from build123d import *

# Parameters (mm, degrees)
BOSS_EXTRUDE1_DEPTH = 55
SKETCH2_R           = 2.5
CUT_EXTRUDE1_DEPTH  = 2
SKETCH3_W           = 1
SKETCH3_H           = 9
CUT_EXTRUDE2_DEPTH  = 35
SKETCH4_R           = 2.25
CUT_EXTRUDE3_DEPTH  = 11


with BuildPart() as part:
    # Sketch1 → Boss-Extrude1 (new body)
    with BuildSketch(Plane.XY):
        Polygon((0, 10), (0, 0), (10, 0), (10, 1), (1, 1), (1, 10), align=None)
    extrude(amount=BOSS_EXTRUDE1_DEPTH)

    # Sketch2 → Cut-Extrude1 (cut, through all)
    with BuildSketch(Plane(origin=(0, 1, 0), x_dir=(1, 0, 0), z_dir=(0, 1, 0))):
        with Locations((5, -50)):
            Circle(SKETCH2_R)
        with Locations((5, -26.95)):
            Circle(SKETCH2_R)
        with BuildLine():
            Line((-2.7555139, -28.141028133), (-2.7555139, -48.808971867))
            ThreePointArc((-2.7555139, -48.808971867), (4.475, -38.475), (-2.7555139, -28.141028133))
        make_face()
    extrude(amount=-CUT_EXTRUDE1_DEPTH, mode=Mode.SUBTRACT)

    # Sketch3 → Cut-Extrude2 (cut)
    with BuildSketch(Plane.XY.offset(55)):
        with Locations((0.5, 5.5)):
            Rectangle(SKETCH3_W, SKETCH3_H)
    extrude(amount=-CUT_EXTRUDE2_DEPTH, mode=Mode.SUBTRACT)

    # Sketch4 → Cut-Extrude3 (cut, through all)
    with BuildSketch(Plane.ZY):
        with Locations((5.1, 4)):
            Circle(SKETCH4_R)
        with Locations((15.1, 4)):
            Circle(SKETCH4_R)
    extrude(amount=-CUT_EXTRUDE3_DEPTH, mode=Mode.SUBTRACT)


solid = part.part
The model under review builds one solid part; all positions refer to its coordinate system, in mm. A direction names the side the tool comes from. Round coordinates to 2 decimals unless told otherwise and drop trailing zeros. Loops run counter-clockwise (first coordinate to the right, second up) from the corner with the lowest first, then second, coordinate; pieces in that order, holes last. Notation, with made-up numbers: M 51.5,-1 L 69.5,-1 A19 cw 69.5,13 Z; hole C 72,33.5 d8. An arc over 180 degrees is marked long. Answer as CSV lines item,"result". Start each with the question number.
Item 1: Wall thickness on line 1 (X direction, y = 0.3, z = 26.95); line 2 (Z direction, x = 5, y = 0.55); line 3 (Y direction, x = 0.4, z = 5.1): over which ranges is each line inside the solid? List them lowest first. Write a range as [from, to].
Item 2: Consider section A-A (x = 5). Write out the cut boundary in (y, z).
Item 3: Insertion check: P1, Ø4.5, axis at x = 5, z = 50, coming from the -Y side; P2, Ø1.1, axis at x = 0.5, y = 6, coming from the +Z side. Each pin has a flat end and moves straight along its axis. Give the tip position at first contact, or say it passes through.
Item 4: Consider section B-B (z = 50). Write out the cut boundary in (x, y), then the cut area to 3 significant figures.
Item 5: For faces 4 (the face through (1, 5, 10)), 5 (the face through (0.5, 5.6, 20)), 6 (the face through (5, 0, 21)), list the 3-axis set-ups (+Z, -Z, +X, -X, +Y, -Y) from which the entire face can be reached by the end or side of a thin tool; tool diameter is ignored.
Item 6: Mouldability with a two-part tool opening along X and no side actions: class faces 1 (the face through (4.474, 0.507, 38.619)), 2 (the face through (6.15, 0.51, 29.17)), 3 (the face through (0.493, 4.676, 17.246)) as released by +X, released by -X, zero draft, split by the parting line, or undercut.
Item 7: Consider section D-D (x = 2). Write out the cut boundary in (y, z), then the cut area to 3 significant figures.
Item 8: Consider section C-C (y = 4). Write out the cut boundary in (x, z).
Answer:
1,line 1,"x = [0, 2.5], [7.5, 10]"
1,line 2,"z = [0, 24.45], [29.45, 47.5], [52.5, 55]"
1,line 3,"y = [0, 1.75], [6.25, 10]"
2,outline,"M 0,0 L 1,0 L 1,24.45 L 0,24.45 Z; M 0,29.45 L 1,29.45 L 1,47.5 L 0,47.5 Z; M 0,52.5 L 1,52.5 L 1,55 L 0,55 Z"
3,P1,"passes through"
3,P2,"stops at z = 20"
4,outline,"M 0,0 L 2.5,0 L 2.5,1 L 0,1 Z; M 7.5,0 L 10,0 L 10,1 L 7.5,1 Z"
4,area,"5.00 mm^2"
5,face 4,"+Z, -Z, +X, +Y"
5,face 5,"+Z, +X, -X, +Y"
5,face 6,"+Z, -Z, +X, -X, -Y"
6,face 1,"released by -X"
6,face 2,"undercut"
6,face 3,"zero draft"
7,outline,"M 0,0 L 1,0 L 1,31.52 L 0,31.52 Z; M 0,45.43 L 1,45.43 L 1,55 L 0,55 Z"
7,area,"41.1 mm^2"
8,outline,"M 0,0 L 1,0 L 1,2.85 L 0,2.85 Z; M 0,7.35 L 1,7.35 L 1,12.85 L 0,12.85 Z; M 0,17.35 L 1,17.35 L 1,20 L 0,20 Z"
